Work out the finished part from the listing and answer in its coordinate system (mm). A direction names the side the tool comes from. Coordinates: 2 decimals unless noted, no trailing zeros. Order: outer loops, then holes, each group sorted by start corner. A loop starts at its lowest first (then second) coordinate and runs counter-clockwise, first axis right, second up. Notation, with made-up numbers: (44, 15.5) -> (59, 15.5) arc R12 cw to (59, 32.5) -> close; hole circle Ø7 at (-13.75, 83). An arc over 180 degrees is marked (long way). Write item = value, one per line. Start each with the question number.
Q1. Which of the six approach directions +Z, -Z, +X, -X, +Y, -Y give full straight-line access (tool end or side, diameter ignored) to faces 1 (the flat face through (-35, -20, -19)), 2 (the flat face through (-33, 16, -8)), 3 (the flat face through (-35, 20, -1))?
Q2. For a pull along Z with two mould halves and no side action, classify faces 4 (the flat face through (-35, -20, -1)), 5 (the cylindrical face through (-36, 21, -10)), 6 (the flat face through (-37, 30, -10)), 7 (the cylindrical face through (-35.96, -16.39, -11.34)) as +Z half, -Z half, draft (parallel to the pull), parting line (faces both ways), or undercut.
Q3. Flat-ended cylindrical pins translate along their axes: pin 1 (7 mm diameter, centred on y = 18.5, z = -11, fed in from +X); pin 2 (3 mm diameter, centred on x = 2, z = -5.5, fed in from -Y); pin 3 (6 mm diameter, centred on x = 23.5, z = -9.5, fed in from +Y). Find the tip coordinate at first contact, or state that the pin passes through.
Q4. Straight lines are drawn through the part: L1, parallel to Y at x = -36.2, z = -10; L2, parallel to Y at x = -35.8, z = -10; L3, parallel to Z at x = -37.7, y = 18.5. For each, find the intervals that lie inside material, in ascending order. Write a range as from..to.
Q5. The part is cut by section A-A, the plane z = -10. Determine the outline of the cut face in (x, y).
Q6. The part is cut by section B-B, the plane y = 18.5. Determine the outline of the cut face in (x, z), plus the area to 3 significant figures.
Q7. The part is cut by section C-C, the plane y = -12. Determine the outline of the cut face in (x, z).
Q8. The part is cut by section D-D, the plane z = -6.25. Determine the outline of the cut face in (x, y), plus the area to 3 significant figures.
Solid Edge part; units mm, degrees
sketch "Sketch1" plane through (0, 0, 0) normal (0, 0, 1) x (1, 0, 0)
  line L0 (33, -10) -> (33, 10)
  line L1 (33, 10) -> (-33, 10)
  line L2 (-33, 10) -> (-33, 30)
  line L3 (-33, 30) -> (-39, 30)
  line L4 (-39, -30) -> (-39, 30)
  line L5 (-33, -30) -> (-39, -30)
  line L6 (-33, -10) -> (-33, -30)
  line L7 (-33, -10) -> (33, -10)
extrude "Protrusion1" add sketch "Sketch1" against normal blind 20
chamfer "Chanfro_1" distance 3 angle 45 6 edges at (-33, -20, -20) (-33, -30, -10) (-33, -20, 0) (-33, 20, -20) (-33, 30, -10) (-33, 20, 0)
hole "Furo_3" at (-33, 18.5, -10) direction (-1, 0, 0) diameter 5 end up to next
hole "Hole1" at (-33, -18.5, -10) direction (-1, 0, 0) diameter 5 end up to next
Model answer:
q1.face_1 = -Z, +X, -Y
q1.face_2 = +Z, -Z, +X, +Y
q1.face_3 = +Z, +X, +Y
q2.face_4 = +Z half
q2.face_5 = undercut
q2.face_6 = draft
q2.face_7 = undercut
q3.pin_1 = -33
q3.pin_2 = -10
q3.pin_3 = 10
q4.L1 = -30..-21, -16..16, 21..30
q4.L2 = -29.8..-21, -16..16, 21..29.8
q4.L3 = -20..-12.5, -7.5..0
q5.outline = (-39, -30) -> (-36, -30) -> (-33, -27) -> (-33, -21) -> (-39, -21) -> close; (-39, -16) -> (-33, -16) -> (-33, -10) -> (33, -10) -> (33, 10) -> (-33, 10) -> (-33, 16) -> (-39, 16) -> close; (-39, 21) -> (-33, 21) -> (-33, 27) -> (-36, 30) -> (-39, 30) -> close
q6.outline = (-39, -20) -> (-36, -20) -> (-33, -17) -> (-33, -12.5) -> (-39, -12.5) -> close; (-39, -7.5) -> (-33, -7.5) -> (-33, -3) -> (-36, 0) -> (-39, 0) -> close
q6.area = 81.0 mm2
q7.outline = (-39, -20) -> (-36, -20) -> (-33, -17) -> (-33, -3) -> (-36, 0) -> (-39, 0) -> close
q8.outline = (-39, -30) -> (-36, -30) -> (-33, -27) -> (-33, -10) -> (33, -10) -> (33, 10) -> (-33, 10) -> (-33, 27) -> (-36, 30) -> (-39, 30) -> close
q8.area = 1,670 mm2
